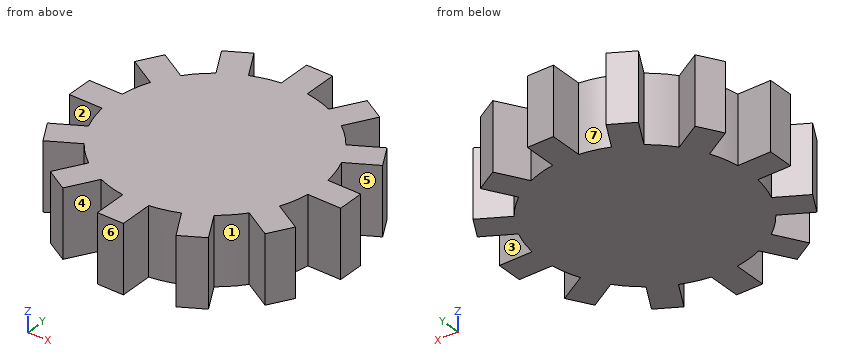
```python
from build123d import *

# Parameters (mm, degrees)
F1_DEPTH = 15


with BuildPart() as f1:
    # F0 (on Top) → F1 (new body)
    with BuildSketch(Plane.XY):
        with BuildLine():
            Line((-2.888783, 30.191496), (-2.888783, 22.877379))
            ThreePointArc((-2.888783, 22.877379), (-5.96812, 22.273326), (-8.93693, 21.256782))
            Line((-8.93693, 21.256782), (-12.593989, 27.590994))
            Line((-12.593989, 27.590994), (-17.597507, 24.702211))
            Line((-17.597507, 24.702211), (-13.940448, 18.368))
            ThreePointArc((-13.940448, 18.368), (-16.305207, 16.305207), (-18.368, 13.940448))
            Line((-18.368, 13.940448), (-24.702211, 17.597507))
            Line((-24.702211, 17.597507), (-27.590994, 12.593989))
            Line((-27.590994, 12.593989), (-21.256782, 8.93693))
            ThreePointArc((-21.256782, 8.93693), (-22.273326, 5.96812), (-22.877379, 2.888783))
            Line((-22.877379, 2.888783), (-30.191496, 2.888783))
            Line((-30.191496, 2.888783), (-30.191496, -2.888783))
            Line((-30.191496, -2.888783), (-22.877379, -2.888783))
            ThreePointArc((-22.877379, -2.888783), (-22.273326, -5.96812), (-21.256782, -8.93693))
            Line((-21.256782, -8.93693), (-27.590994, -12.593989))
            Line((-27.590994, -12.593989), (-24.702211, -17.597507))
            Line((-24.702211, -17.597507), (-18.368, -13.940448))
            ThreePointArc((-18.368, -13.940448), (-16.305207, -16.305207), (-13.940448, -18.368))
            Line((-13.940448, -18.368), (-17.597507, -24.702211))
            Line((-17.597507, -24.702211), (-12.593989, -27.590994))
            Line((-12.593989, -27.590994), (-8.93693, -21.256782))
            ThreePointArc((-8.93693, -21.256782), (-5.96812, -22.273326), (-2.888783, -22.877379))
            Line((-2.888783, -22.877379), (-2.888783, -30.191496))
            Line((-2.888783, -30.191496), (2.888783, -30.191496))
            Line((2.888783, -30.191496), (2.888783, -22.877379))
            ThreePointArc((2.888783, -22.877379), (5.96812, -22.273326), (8.93693, -21.256782))
            Line((8.93693, -21.256782), (12.593989, -27.590994))
            Line((12.593989, -27.590994), (17.597507, -24.702211))
            Line((17.597507, -24.702211), (13.940448, -18.368))
            ThreePointArc((13.940448, -18.368), (16.305207, -16.305207), (18.368, -13.940448))
            Line((18.368, -13.940448), (24.702211, -17.597507))
            Line((24.702211, -17.597507), (27.590994, -12.593989))
            Line((27.590994, -12.593989), (21.256782, -8.93693))
            ThreePointArc((21.256782, -8.93693), (22.273326, -5.96812), (22.877379, -2.888783))
            Line((22.877379, -2.888783), (30.191496, -2.888783))
            Line((30.191496, -2.888783), (30.191496, 2.888783))
            Line((30.191496, 2.888783), (22.877379, 2.888783))
            ThreePointArc((22.877379, 2.888783), (22.273326, 5.96812), (21.256782, 8.93693))
            Line((21.256782, 8.93693), (27.590994, 12.593989))
            Line((27.590994, 12.593989), (24.702211, 17.597507))
            Line((24.702211, 17.597507), (18.368, 13.940448))
            ThreePointArc((18.368, 13.940448), (16.305207, 16.305207), (13.940448, 18.368))
            Line((13.940448, 18.368), (17.597507, 24.702211))
            Line((17.597507, 24.702211), (12.593989, 27.590994))
            Line((12.593989, 27.590994), (8.93693, 21.256782))
            ThreePointArc((8.93693, 21.256782), (5.96812, 22.273326), (2.888783, 22.877379))
            Line((2.888783, 22.877379), (2.888783, 30.191496))
            Line((2.888783, 30.191496), (-2.888783, 30.191496))
        make_face()
    extrude(amount=F1_DEPTH)


solid = f1.part
```
Input: part model. Units: mm. Frame: model coordinates. Face numbers are marked on the shaded views. A direction names the side the tool comes from. Give positions to 0.01 mm unless a question says otherwise; leave off trailing zeros. Order: outer loops, then holes, each group sorted by start corner. A loop starts at its lowest first (then second) coordinate and runs counter-clockwise, first axis right, second up. Notation, with made-up numbers: (67, -20) - (115, -20) arc R32 ccw to (115, 7) - close; hole circle Ø11 at (85.25, 58). An arc over 180 degrees is marked (long way). Use a Markdown table: item, result.
(1) Access query for the marked faces 1, 2, 3 and 4. Directions: +Z, -Z, +X, -X, +Y, -Y. A direction counts if a zero-diameter tool reaches every point of the face in a straight line with its end or side. Return the directions, or none.
Computed values:
| item | result |
|---|---|
| face 1 | +Z, -Z |
| face 2 | +Z, -Z, -X |
| face 3 | +Z, -Z, +X |
| face 4 | +Z, -Z, -Y |
(2) Pin query (flat end, axial travel): pin 1 (12 mm diameter, centred on x = 3, y = 10, fed in from -Z); pin 2 (2 mm diameter, centred on y = 27.5, z = 7, fed in from +X); pin 3 (4 mm diameter, centred on x = 10, z = 6.5, fed in from +Y); pin 4 (6 mm diameter, centred on x = 28, z = 7, fed in from +Y). Return the tip coordinate at first contact, or that it passes through.
Computed values:
| item | result |
|---|---|
| pin 1 | stops at z = 0 |
| pin 2 | stops at x = 14.48 |
| pin 3 | stops at y = 26.56 |
| pin 4 | stops at y = 17.08 |
(3) Section query B-B (y = 26.5). Output: boundary loops of the cut face in (x, z).
Computed values:
| item | result |
|---|---|
| outline | (-14.48, 0) - (-11.96, 0) - (-11.96, 15) - (-14.48, 15) - close; (-2.89, 0) - (2.89, 0) - (2.89, 15) - (-2.89, 15) - close; (11.96, 0) - (14.48, 0) - (14.48, 15) - (11.96, 15) - close |
(4) Section query D-D (x = 8). Output: boundary loops of the cut face in (y, z), then the cut area to 3 significant figures.
Computed values:
| item | result |
|---|---|
| outline | (-21.63, 0) - (21.63, 0) - (21.63, 15) - (-21.63, 15) - close |
| area | 649 mm2 |
(5) Section query A-A (x = 24). Output: boundary loops of the cut face in (y, z).
Computed values:
| item | result |
|---|---|
| outline | (-17.19, 0) - (-10.52, 0) - (-10.52, 15) - (-17.19, 15) - close; (-2.89, 0) - (2.89, 0) - (2.89, 15) - (-2.89, 15) - close; (10.52, 0) - (17.19, 0) - (17.19, 15) - (10.52, 15) - close |
(6) Section query C-C (y = -6). Output: boundary loops of the cut face in (x, z).
Computed values:
| item | result |
|---|---|
| outline | (-22.26, 0) - (22.26, 0) - (22.26, 15) - (-22.26, 15) - close |
(7) Draft query along X for the marked faces 5, 6 and 7. Return one class per face: released by +X, released by -X, zero draft, split by the parting line, or undercut.
Computed values:
| item | result |
|---|---|
| face 5 | released by +X |
| face 6 | zero draft |
| face 7 | undercut |
(8) Line query: line 1 (X direction, y = 16.5, z = 3); line 2 (X direction, y = 17, z = 6); line 3 (Y direction, x = -25.5, z = 3.75). Output: solid intervals per line, ascending. Write a range as from..to.
Computed values:
| item | result |
|---|---|
| line 1 | x = -25.34..-22.8, -16.11..16.11, 22.8..25.34 |
| line 2 | x = -25.05..-23.67, -15.58..15.58, 23.67..25.05 |
| line 3 | y = -16.22..-11.39, -2.89..2.89, 11.39..16.22 |
